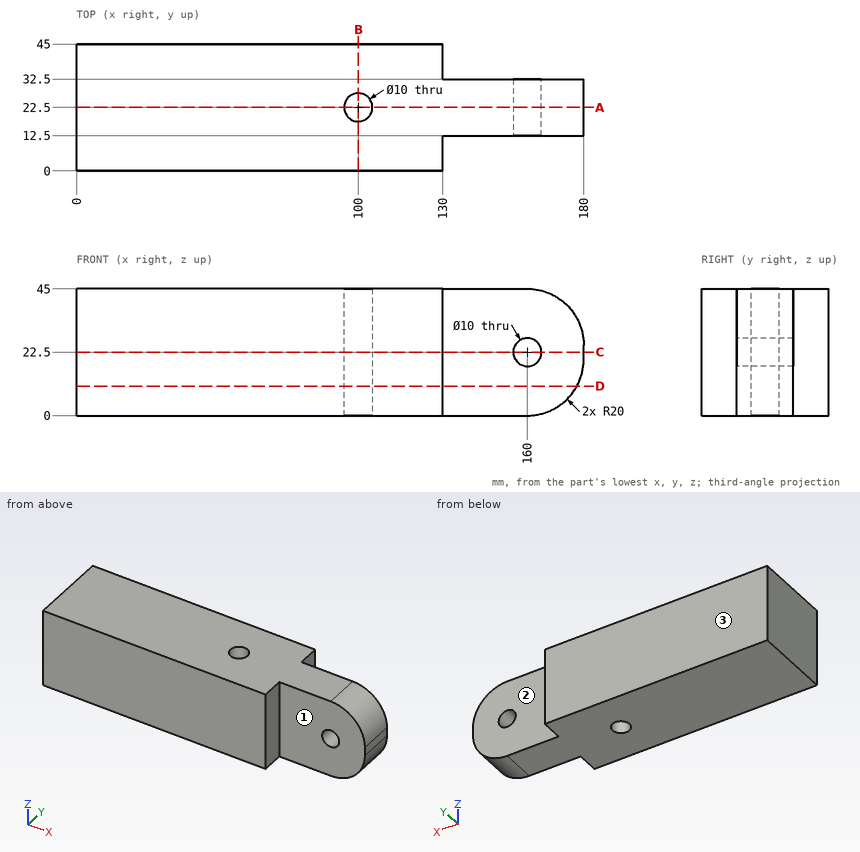
Here's the drawing with two shaded views (mm, measured from the low corner). I have some questions. A direction names the side the tool comes from. Give positions to 0.01 mm unless a question says otherwise; leave off trailing zeros. Order: outer loops, then holes, each group sorted by start corner. A loop starts at its lowest first (then second) coordinate and runs counter-clockwise, first axis right, second up. Notation, with made-up numbers: M 6.25,-2.75 L 49.25,-2.75 A30 ccw 49.25,32.25 Z; hole C -4.75,72 d5. An arc over 180 degrees is marked long. Answer as a JSON object with one key per item and string values. Group by question number.
1) Suppose I cut it at B-B, the plane x = 100. Write out the boundary of the cut face in (y, z), plus the area to 4 significant figures.
2) On a 3-axis mill with a long thin cutter (end or side, diameter ignored), from which of +Z, -Z, +X, -X, +Y, -Y can I reach the whole of each face in a straight line? I mean the marked faces 1, 2 and 3. Say none if no direction works.
3) Please list where these lines run through material, in increasing order: L1, parallel to Z at x = 160, y = 27; L2, parallel to X at y = 18, z = 38. Write a range as [from, to].
4) I'm going to push flat-ended pins straight in: pin 1 Ø6 at (y, z) = (7.5, 24) entering from +X; pin 2 Ø5 at (y, z) = (27, 5) entering from +X; pin 3 Ø1.5 at (x, z) = (96, 14) entering from -Y; pin 4 Ø16 at (x, z) = (160, 22.5) entering from +Y. Where does each tip first touch, or does it pass through?
5) Suppose I cut it at C-C, the plane z = 22.5. Write out the boundary of the cut face in (x, y), plus the area to 3 significant figures.
6) Suppose I cut it at D-D, the plane z = 10.5. Write out the boundary of the cut face in (x, y), plus the area to 3 significant figures.
7) Suppose I cut it at A-A, the plane y = 22.5. Write out the boundary of the cut face in (x, z).
Results found:
{
 "1": {"outline": "M 0,0 L 17.5,0 L 17.5,45 L 0,45 Z; M 27.5,0 L 45,0 L 45,45 L 27.5,45 Z", "area": "1,575 mm²"},
 "2": {"face 1": "+Z, -Z, +X, -Y", "face 2": "+Z, -Z, +X, +Y", "face 3": "+Z, -Z, +X, -X, +Y"},
 "3": {"L1": "[0, 17.5], [27.5, 45]", "L2": "[0, 97.82], [102.18, 175.2]"},
 "4": {"pin 1": "x = 130", "pin 2": "x = 175.61", "pin 3": "y = 0", "pin 4": "y = 32.5"},
 "5": {"outline": "M 0,0 L 130,0 L 130,12.5 L 155,12.5 L 155,32.5 L 130,32.5 L 130,45 L 0,45 Z; M 165,12.5 L 180,12.5 L 180,32.5 L 165,32.5 Z; hole C 100,22.5 d10", "area": "6,570 mm²"},
 "6": {"outline": "M 0,0 L 130,0 L 130,12.5 L 177.6,12.5 L 177.6,32.5 L 130,32.5 L 130,45 L 0,45 Z; hole C 100,22.5 d10", "area": "6,720 mm²"},
 "7": {"outline": "M 0,0 L 95,0 L 95,45 L 0,45 Z; M 105,0 L 160,0 A20 ccw 180,20 L 180,25 A20 ccw 160,45 L 105,45 Z; hole C 160,22.5 d10"}
}
